The listing builds one solid part. Answer for the finished solid, in the listing's coordinates (mm). Give positions to 0.01 mm unless a question says otherwise; leave off trailing zeros. Order: outer loops, then holes, each group sorted by start corner. A loop starts at its lowest first (then second) coordinate and runs counter-clockwise, first axis right, second up. Notation, with made-up numbers: (86.25, 87.25) - (144.25, 87.25) arc R31 cw to (144.25, 122.25) - close; hole circle Ø11 at (54, -20). An arc over 180 degrees is marked (long way). Answer as a JSON object with one key per item and string values. Group by question number.
Q1. A cutting plane is placed at C-C, the plane x = -29.5. Give the vertices of the cut face in (y, z), and give its area (3 significant figures).
Q2. A cutting plane is placed at B-B, the plane y = -4. Give the vertices of the cut face in (x, z), and give its area (3 significant figures).
Q3. Consider line 1 (Y direction, x = -25, z = 0.85); line 2 (X direction, y = 0.5, z = 2.5); line 3 (Y direction, x = 29, z = 1.7). Determine where each line is inside the solid, lowest interval first.
Q4. A cutting plane is placed at A-A, the plane z = 1.9. Count the separate pieces of the cut face and the enclosed holes in it, and give its area (3 significant figures).
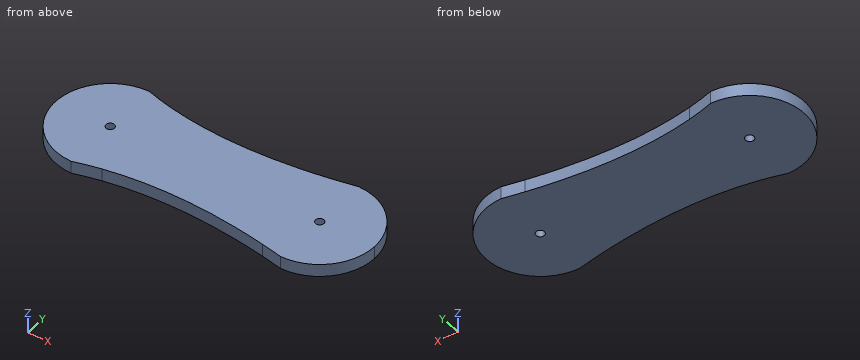
from build123d import *

# Parameters (mm, degrees)
SKETCH1_R           = 1
BOSS_EXTRUDE1_DEPTH = 3


with BuildPart() as part:
    # Sketch1 → Boss-Extrude1 (new body)
    # profile 1 of 6: a face of its own
    with BuildSketch(Plane.XY):
        with BuildLine():
            ThreePointArc((-24.781290204, -3.3929583), (-28.4, 0), (-24.781290204, 3.3929583))
            Line((-24.781290204, 3.3929583), (-12.188441083, 2.581224344))
            ThreePointArc((-12.188441083, 2.581224344), (-14.492522891, 7.771208774), (-18.780288742, 11.494083385))
            add(Edge.make_bspline(
                [(-25, 13.069), (-21.982355601, 12.146946089), (-18.780288742, 11.494083385)],
                knots=[0, 0, 0, 0.145973682, 0.145973682, 0.145973682], degree=2))
            ThreePointArc((-25, 13.069), (-38.069, 0), (-25, -13.069))
            add(Edge.make_bspline(
                [(-25, -13.069), (-21.982355601, -12.146946089), (-18.780288742, -11.494083385)],
                knots=[0, 0, 0, 0.145973682, 0.145973682, 0.145973682], degree=2))
            ThreePointArc((-18.780288742, -11.494083385), (-14.492522891, -7.771208774), (-12.188441083, -2.581224344))
            Line((-12.188441083, -2.581224344), (-24.781290204, -3.3929583))
        make_face()
    # profile 2 of 6: a face of its own
    with BuildSketch(Plane.XY):
        with BuildLine():
            ThreePointArc((-18.780288742, 11.494083385), (-14.492522891, 7.771208774), (-12.188441083, 2.581224344))
            Line((-12.188441083, 2.581224344), (-3.107347179, 1.995857823))
            ThreePointArc((-3.107347179, 1.995857823), (-1.236, 0), (-3.107347179, -1.995857823))
            Line((-3.107347179, -1.995857823), (-12.188441083, -2.581224344))
            ThreePointArc((-12.188441083, -2.581224344), (-14.492522891, -7.771208774), (-18.780288742, -11.494083385))
            add(Edge.make_bspline(
                [(-18.780288742, -11.494083385), (-1.944343038, -8.061437688), (19.989933944, -12.070542619)],
                knots=[0.145973682, 0.145973682, 0.145973682, 0.91347951, 0.91347951, 0.91347951], degree=2))
            ThreePointArc((19.989933944, -12.070542619), (14.904735293, -8.299662132), (12.188441083, -2.581224344))
            Line((12.188441083, -2.581224344), (3.107347179, -1.995857823))
            ThreePointArc((3.107347179, -1.995857823), (1.236, 0), (3.107347179, 1.995857823))
            Line((3.107347179, 1.995857823), (12.188441083, 2.581224344))
            ThreePointArc((12.188441083, 2.581224344), (14.904735293, 8.299662132), (19.989933944, 12.070542619))
            add(Edge.make_bspline(
                [(-18.780288742, 11.494083385), (-1.944343038, 8.061437688), (19.989933944, 12.070542619)],
                knots=[0.145973682, 0.145973682, 0.145973682, 0.91347951, 0.91347951, 0.91347951], degree=2))
        make_face()
    # profile 3 of 6: a face of its own
    with BuildSketch(Plane.XY):
        with BuildLine():
            add(Edge.make_bspline(
                [(19.989933944, 12.070542619), (22.462572371, 12.522486712), (25, 13.069)],
                knots=[0.91347951, 0.91347951, 0.91347951, 1, 1, 1], degree=2))
            ThreePointArc((19.989933944, 12.070542619), (14.904735293, 8.299662132), (12.188441083, 2.581224344))
            Line((12.188441083, 2.581224344), (24.781290204, 3.3929583))
            ThreePointArc((24.781290204, 3.3929583), (28.4, 0), (24.781290204, -3.3929583))
            Line((24.781290204, -3.3929583), (12.188441083, -2.581224344))
            ThreePointArc((12.188441083, -2.581224344), (14.904735293, -8.299662132), (19.989933944, -12.070542619))
            add(Edge.make_bspline(
                [(19.989933944, -12.070542619), (22.462572371, -12.522486712), (25, -13.069)],
                knots=[0.91347951, 0.91347951, 0.91347951, 1, 1, 1], degree=2))
            ThreePointArc((25, -13.069), (34.241178523, -9.241178523), (38.069, 0))
            ThreePointArc((38.069, 0), (34.241178523, 9.241178523), (25, 13.069))
        make_face()
    # profile 4 of 6: a face of its own
    with BuildSketch(Plane.XY):
        with BuildLine():
            Line((24.781290204, 3.3929583), (12.188441083, 2.581224344))
            ThreePointArc((12.188441083, 2.581224344), (11.931, 0), (12.188441083, -2.581224344))
            Line((12.188441083, -2.581224344), (24.781290204, -3.3929583))
            ThreePointArc((24.781290204, -3.3929583), (28.4, 0), (24.781290204, 3.3929583))
        make_face()
        with Locations((25, 0)):
            Circle(SKETCH1_R, mode=Mode.SUBTRACT)
    # profile 5 of 6: a face of its own
    with BuildSketch(Plane.XY):
        with BuildLine():
            ThreePointArc((12.188441083, -2.581224344), (11.931, 0), (12.188441083, 2.581224344))
            Line((12.188441083, 2.581224344), (3.107347179, 1.995857823))
            ThreePointArc((3.107347179, 1.995857823), (1.236, 0), (3.107347179, -1.995857823))
            Line((3.107347179, -1.995857823), (12.188441083, -2.581224344))
        make_face()
    # profile 6 of 6: a face of its own
    with BuildSketch(Plane.XY):
        with BuildLine():
            Line((-24.781290204, -3.3929583), (-3.107347179, -1.995857823))
            ThreePointArc((-3.107347179, -1.995857823), (-1.236, 0), (-3.107347179, 1.995857823))
            Line((-3.107347179, 1.995857823), (-24.781290204, 3.3929583))
            ThreePointArc((-24.781290204, 3.3929583), (-28.4, 0), (-24.781290204, -3.3929583))
        make_face()
        with Locations((-25, 0)):
            Circle(SKETCH1_R, mode=Mode.SUBTRACT)
    extrude(amount=BOSS_EXTRUDE1_DEPTH)


solid = part.part
Reply:
{
 "1": {"outline": "(-12.27, 0) - (12.27, 0) - (12.27, 3) - (-12.27, 3) - close", "area": "73.6 mm^2"},
 "2": {"outline": "(-37.44, 0) - (37.44, 0) - (37.44, 3) - (-37.44, 3) - close", "area": "225 mm^2"},
 "3": {"line 1": "y = -13.07 to -1, 1 to 13.07", "line 2": "x = -38.06 to -25.87, -24.13 to 24.13, 25.87 to 38.06", "line 3": "y = -12.44 to 12.44"},
 "4": {"separate pieces": "1", "enclosed holes": "2", "area": "1,630 mm^2"}
}
